```python
from build123d import *

# Parameters (mm, degrees)
SKETCH1_W           = 120
SKETCH1_H           = 90
BOSS_EXTRUDE1_DEPTH = 3
SKETCH2_R           = 1.75
CUT_EXTRUDE1_DEPTH  = 3
CUT_EXTRUDE2_DEPTH  = 3


with BuildPart() as part:
    # Sketch1 → Boss-Extrude1 (new body)
    with BuildSketch(Plane.XY):
        with Locations((60, -45)):
            Rectangle(SKETCH1_W, SKETCH1_H)
    extrude(amount=BOSS_EXTRUDE1_DEPTH)

    # Sketch2 → Cut-Extrude1 (cut)
    with BuildSketch(Plane.XY.offset(3)):
        with Locations((24, -44.9)):
            Circle(SKETCH2_R)
    extrude(amount=-CUT_EXTRUDE1_DEPTH, mode=Mode.SUBTRACT)

    # Sketch3 → Cut-Extrude2 (cut)
    with BuildSketch(Plane.XY.offset(3)):
        with BuildLine():
            Line((19, -84.65), (39, -84.65))
            ThreePointArc((39, -84.65), (40.35, -86), (39, -87.35))
            Line((39, -87.35), (19, -87.35))
            ThreePointArc((19, -87.35), (17.65, -86), (19, -84.65))
        make_face()
    extrude(amount=-CUT_EXTRUDE2_DEPTH, mode=Mode.SUBTRACT)


solid = part.part
```
Design review of the part built by this model. Coordinates are the model's own, in mm. A direction names the side the tool comes from. Give positions to 0.01 mm unless a question says otherwise; leave off trailing zeros. Order: outer loops, then holes, each group sorted by start corner. A loop starts at its lowest first (then second) coordinate and runs counter-clockwise, first axis right, second up. Notation, with made-up numbers: (44, -33) -> (58, -33) arc R13 ccw to (58, -12) -> close; hole circle Ø4 at (-23.75, 6). An arc over 180 degrees is marked (long way). Write item = value, one per line. Start each with the question number.
(1) We need section C-C on y = -86. Write out the cut boundary in (x, z).
(2) For faces 1 (the face through (29, -87.35, 2)), 2 (the face through (59, -44, 3)), list the 3-axis set-ups (+Z, -Z, +X, -X, +Y, -Y) from which the entire face can be reached by the end or side of a thin tool; tool diameter is ignored.
(3) We need section B-B on y = -44.9. Write out the cut boundary in (x, z).
(4) Mouldability with a two-part tool opening along X and no side actions: class faces 3 (the face through (0, -46, 1)), 4 (the face through (17.65, -86.03, 1.52)), 5 (the face through (59, -44, 0)) as +X half, -X half, draft (parallel to the pull), parting line (faces both ways), or undercut.
(5) We need section A-A on x = 24. Write out the cut boundary in (y, z), plus the area to 3 significant figures.
(6) For pin 1 (2 mm diameter, centred on x = 24, y = -44.9, fed in from -Z), flat-tipped, find the tip position at first contact; note if it passes through.
(7) To check wall thickness, follow line 1 along Y through (x, z) = (24, 2.4); line 2 along Y through (x, z) = (33.5, 1.55); line 3 along X through (y, z) = (-45.5, 2.8). State the ranges of each line that lie inside material, in increasing order.
Numbers:
q1.outline = (0, 0) -> (17.65, 0) -> (17.65, 3) -> (0, 3) -> close; (40.35, 0) -> (120, 0) -> (120, 3) -> (40.35, 3) -> close
q2.face_1 = +Z, -Z
q2.face_2 = +Z, +X, -X, +Y, -Y
q3.outline = (0, 0) -> (22.25, 0) -> (22.25, 3) -> (0, 3) -> close; (25.75, 0) -> (120, 0) -> (120, 3) -> (25.75, 3) -> close
q4.face_3 = -X half
q4.face_4 = undercut
q4.face_5 = draft
q5.outline = (-90, 0) -> (-87.35, 0) -> (-87.35, 3) -> (-90, 3) -> close; (-84.65, 0) -> (-46.65, 0) -> (-46.65, 3) -> (-84.65, 3) -> close; (-43.15, 0) -> (0, 0) -> (0, 3) -> (-43.15, 3) -> close
q5.area = 251 mm^2
q6.pin_1 = through
q7.line_1 = -90 to -87.35, -84.65 to -46.65, -43.15 to 0
q7.line_2 = -90 to -87.35, -84.65 to 0
q7.line_3 = 0 to 22.36, 25.64 to 120
